Could you check a few things on this model? Use its own coordinates, in mm. Face numbers are marked on the shaded views. A direction names the side the tool comes from. Give positions to 0.01 mm unless a question says otherwise; leave off trailing zeros. Loops run counter-clockwise (first coordinate to the right, second up) from the corner with the lowest first, then second, coordinate; pieces in that order, holes last. Notation, with made-up numbers: (58.25, 26.25) -> (108.25, 26.25) arc R29 cw to (108.25, 58.25) -> close; hole circle Ø5 at (70, 82). An arc over 180 degrees is marked (long way). Write item = value, one per line. Start each with the question number.
1) I want a section at D-D (z = -36). List the corners of the cut face in (x, y) for me.
2) I want a section at B-B (x = -100). List the corners of the cut face in (y, z) for me, and give its area (3 significant figures).
3) I need wall thicknesses on probe 1 along X at (y, z) = (18.5, -45.4); probe 2 along Y at (x, z) = (-100, -44.9); probe 3 along Z at (x, y) = (3, 31.5). Which ranges of each line are inside material? Lowest first, please. Write a range as from..to.
4) I want a section at A-A (z = 4). List the corners of the cut face in (x, y) for me.
5) If we mould it in two halves opening along Z, with no side actions, what happens to the marked faces 1, 2, 3 and 4? For each: +Z half, -Z half, draft (parallel to the pull), parting line (faces both ways), or undercut.
6) On a 3-axis mill with a long thin cutter (end or side, diameter ignored), from which of +Z, -Z, +X, -X, +Y, -Y can I reach the whole of each face in a straight line? I mean the marked faces 5, 6 and 7. Say none if no direction works.
7) I'm going to push flat-ended pins straight in: pin 1 Ø12 at (x, z) = (-22.5, -3) entering from +Y; pin 2 Ø12 at (x, z) = (-97.5, 13.5) entering from +Y; pin 3 Ø5 at (x, z) = (-113, 25) entering from -Y. Where does each tip first touch, or does it pass through?
8) I want a section at C-C (y = 63). List the corners of the cut face in (x, z) for me, and give its area (3 significant figures).
from build123d import *

# Parameters (mm, degrees)
SALIENTE_EXTRUIR1_DEPTH    = 47
CROQUIS2_W                 = 50
CROQUIS2_H                 = 38.5
CORTAR_EXTRUIR1_DEPTH      = 281.107568623
SALIENTE_EXTRUIR2_DEPTH    = 3
SALIENTE_EXTRUIR3_DEPTH    = 4
SALIENTE_EXTRUIR4_START    = -4
SALIENTE_EXTRUIR4_DEPTH    = 4
CROQUIS6_W                 = 86
CROQUIS6_H                 = 77
SALIENTE_EXTRUIR5_DEPTH    = 4
CROQUIS7_W                 = 86
CROQUIS7_H                 = 77
SALIENTE_EXTRUIR6_DEPTH    = 4
CORTAR_EXTRUIR2_DEPTH      = 193.353840617
CORTAR_EXTRUIR2_DEPTH_BACK = 193.353840617
CROQUIS9_R                 = 6


with BuildPart() as part:
    # Croquis1 → Saliente-Extruir1 (new, symmetric)
    with BuildSketch(Plane.XY):
        with BuildLine():
            Line((-150, 0), (-120, 0))
            Line((-120, 0), (-120, 18.5))
            ThreePointArc((-120, 18.5), (-100, 38.5), (-80, 18.5))
            Line((-80, 18.5), (-80, 0))
            Line((-80, 0), (80, 0))
            Line((80, 0), (80, 18.5))
            ThreePointArc((80, 18.5), (100, 38.5), (120, 18.5))
            Line((120, 18.5), (120, 0))
            Line((120, 0), (150, 0))
            Line((150, 0), (150, 3))
            Line((150, 3), (123, 3))
            Line((123, 3), (123, 18.5))
            ThreePointArc((123, 18.5), (100, 41.5), (77, 18.5))
            Line((77, 18.5), (77, 3))
            Line((77, 3), (-77, 3))
            Line((-77, 3), (-77, 18.5))
            ThreePointArc((-77, 18.5), (-100, 41.5), (-123, 18.5))
            Line((-123, 18.5), (-123, 3))
            Line((-123, 3), (-150, 3))
            Line((-150, 3), (-150, 0))
        make_face()
    extrude(amount=SALIENTE_EXTRUIR1_DEPTH, both=True)

    # Croquis2 → Cortar-Extruir1 (cut, through all)
    with BuildSketch(Plane(origin=(123, 0, 0), x_dir=(0, 0, -1), z_dir=(1, 0, 0))):
        with Locations((0, 22.25)):
            Rectangle(CROQUIS2_W, CROQUIS2_H)
    extrude(amount=-CORTAR_EXTRUIR1_DEPTH, mode=Mode.SUBTRACT)

    # Croquis3 → Saliente-Extruir2 (add)
    with BuildSketch(Plane.XY.offset(47)):
        with BuildLine():
            Line((120, 18.5), (120, 0))
            Line((120, 0), (80, 0))
            Line((80, 0), (80, 18.5))
            ThreePointArc((80, 18.5), (100, 38.5), (120, 18.5))
        make_face()
        with BuildLine():
            Line((-120, 0), (-120, 18.5))
            ThreePointArc((-120, 18.5), (-100, 38.5), (-80, 18.5))
            Line((-80, 18.5), (-80, 0))
            Line((-80, 0), (-120, 0))
        make_face()
    saliente_extruir2 = extrude(amount=-SALIENTE_EXTRUIR2_DEPTH)

    # Simetría1: Saliente-Extruir2 across plane
    add(saliente_extruir2.mirror(Plane.XY))

    # Croquis4 → Saliente-Extruir3 (add)
    with BuildSketch(Plane.XY.offset(47)):
        with BuildLine():
            Line((150, 80), (-150, 80))
            Line((-150, 80), (-150, 3))
            Line((-150, 3), (-123, 3))
            Line((-123, 3), (-123, 18.5))
            ThreePointArc((-123, 18.5), (-100, 41.5), (-77, 18.5))
            Line((-77, 18.5), (-77, 3))
            Line((-77, 3), (77, 3))
            Line((77, 3), (77, 18.5))
            ThreePointArc((77, 18.5), (100, 41.5), (123, 18.5))
            Line((123, 18.5), (123, 3))
            Line((123, 3), (150, 3))
            Line((150, 3), (150, 80))
        make_face()
    extrude(amount=-SALIENTE_EXTRUIR3_DEPTH)

    # Croquis5 → Saliente-Extruir4 (add)
    with BuildSketch(Plane(origin=(0, 0, -47), x_dir=(-1, 0, 0), z_dir=(0, 0, -1)).offset(SALIENTE_EXTRUIR4_START)):
        with BuildLine():
            Line((123, 3), (150, 3))
            Line((150, 3), (150, 80))
            Line((150, 80), (-150, 80))
            Line((-150, 80), (-150, 3))
            Line((-150, 3), (-123, 3))
            Line((-123, 3), (-123, 18.5))
            ThreePointArc((-123, 18.5), (-100, 41.5), (-77, 18.5))
            Line((-77, 18.5), (-77, 3))
            Line((-77, 3), (77, 3))
            Line((77, 3), (77, 18.5))
            ThreePointArc((77, 18.5), (100, 41.5), (123, 18.5))
            Line((123, 18.5), (123, 3))
        make_face()
    extrude(amount=SALIENTE_EXTRUIR4_DEPTH)

    # Croquis6 → Saliente-Extruir5 (add)
    with BuildSketch(Plane(origin=(150, 0, 0), x_dir=(0, 0, -1), z_dir=(1, 0, 0))):
        with Locations((0, 41.5)):
            Rectangle(CROQUIS6_W, CROQUIS6_H)
    extrude(amount=-SALIENTE_EXTRUIR5_DEPTH)

    # Croquis7 → Saliente-Extruir6 (add)
    with BuildSketch(Plane.ZY.offset(150)):
        with Locations((0, 41.5)):
            Rectangle(CROQUIS7_W, CROQUIS7_H)
    extrude(amount=-SALIENTE_EXTRUIR6_DEPTH)

    # Croquis9 → Cortar-Extruir2 (cut, two sides: drawn at the far end of the back side and taken through both)
    with BuildSketch(Plane(origin=(0, 0, 43), x_dir=(-1, 0, 0), z_dir=(0, 0, -1)).offset(-CORTAR_EXTRUIR2_DEPTH_BACK)):
        with Locations((100, 18.5)):
            Circle(CROQUIS9_R)
        with Locations((-100, 18.5)):
            Circle(CROQUIS9_R)
    extrude(amount=CORTAR_EXTRUIR2_DEPTH + CORTAR_EXTRUIR2_DEPTH_BACK, mode=Mode.SUBTRACT)


solid = part.part
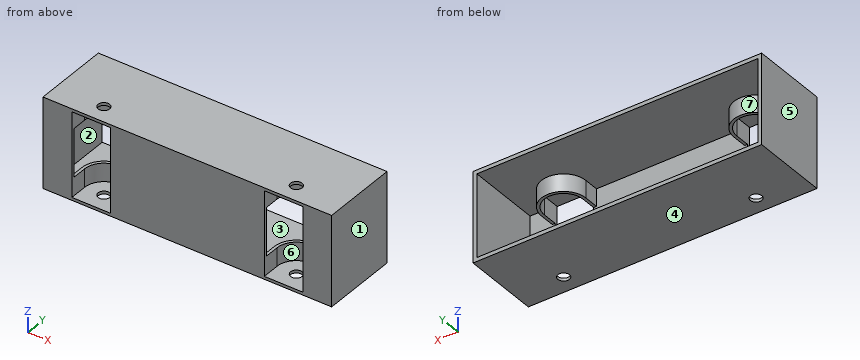
Answer list:
q1.outline = (-150, 0) -> (-120, 0) -> (-120, 18.5) arc R20 cw to (-80, 18.5) -> (-80, 0) -> (80, 0) -> (80, 18.5) arc R20 cw to (120, 18.5) -> (120, 0) -> (150, 0) -> (150, 80) -> (146, 80) -> (146, 3) -> (123, 3) -> (123, 18.5) arc R23 ccw to (77, 18.5) -> (77, 3) -> (-77, 3) -> (-77, 18.5) arc R23 ccw to (-123, 18.5) -> (-123, 3) -> (-146, 3) -> (-146, 80) -> (-150, 80) -> close
q2.outline = (0, -47) -> (12.5, -47) -> (12.5, -44) -> (0, -44) -> close; (0, 44) -> (12.5, 44) -> (12.5, 47) -> (0, 47) -> close; (24.5, -47) -> (80, -47) -> (80, -43) -> (41.5, -43) -> (41.5, -25) -> (38.5, -25) -> (38.5, -44) -> (24.5, -44) -> close; (24.5, 44) -> (38.5, 44) -> (38.5, 25) -> (41.5, 25) -> (41.5, 43) -> (80, 43) -> (80, 47) -> (24.5, 47) -> close
q2.area = 599 mm^2
q3.probe_1 = -150..-106, -94..94, 106..150
q3.probe_2 = 0..12.5, 24.5..80
q3.probe_3 = -47..-43, 43..47
q4.outline = (-150, 0) -> (-120, 0) -> (-120, 3) -> (-146, 3) -> (-146, 80) -> (-150, 80) -> close; (-80, 0) -> (80, 0) -> (80, 3) -> (-80, 3) -> close; (120, 0) -> (150, 0) -> (150, 80) -> (146, 80) -> (146, 3) -> (120, 3) -> close
q5.face_1 = draft
q5.face_2 = undercut
q5.face_3 = undercut
q5.face_4 = -Z half
q6.face_5 = +Z, -Z, -X, +Y, -Y
q6.face_6 = -Y
q6.face_7 = +Y
q7.pin_1 = 3
q7.pin_2 = through
q7.pin_3 = 31.14
q8.outline = (-150, -47) -> (150, -47) -> (150, 47) -> (-150, 47) -> close; hole (-146, -43) -> (146, -43) -> (146, 43) -> (-146, 43) -> close
q8.area = 3,090 mm^2
